Check sheet for the modelled part. Datum: model origin and axes. Units: mm. A direction names the side the tool comes from. Give positions to 0.01 mm unless a question says otherwise; leave off trailing zeros. Write each loop counter-clockwise with the first axis right and the second up, starting at its lowest first coordinate (ties: lowest second). Pieces come first, ordered by that corner, then holes. Notation, with made-up numbers: M 65,-20.75 L 85,-20.75 A21 ccw 85,12.25 Z; hole C 51.25,-20.5 d4. An arc over 180 degrees is marked long. One line per item, written item: value. Start each with the question number.
Autodesk Inventor part; units mm, degrees
ref_plane "Start plane" through (0, 0, 4.5945) normal (0, 0, 1) x (1, 0, 0)
ref_plane "End plane" through (0, 0, 785.2713) normal (0, 0, 1) x (1, 0, 0)
ref_plane "Work Plane4" through (0, 8.5964, 774.6227) normal (0, -0.4912, 0.871) x (1, 0, 0)
ref_plane "Start plane" through (0, 0, 4.5945) normal (0, 0, 1) x (1, 0, 0)
ref_plane "End plane" through (0, 0, 785.2713) normal (0, 0, 1) x (1, 0, 0)
sketch "Sketch" plane through (0, 0, 0) normal (0, 0, 1) x (1, 0, 0)
  line L0 (-17.5, -14.3) -> (-17.5, 14.3)
  line L1 (-14.3, 17.5) -> (14.3, 17.5)
  line L2 (17.5, 14.3) -> (17.5, -14.3)
  line L3 (14.3, -17.5) -> (-14.3, -17.5)
  arc A0 (-17.5, -14.3) -> (-14.3, -17.5) centre (-14.3, -14.3) ccw
  arc A1 (-14.3, 17.5) -> (-17.5, 14.3) centre (-14.3, 14.3) ccw
  arc A2 (17.5, 14.3) -> (14.3, 17.5) centre (14.3, 14.3) ccw
  arc A3 (14.3, -17.5) -> (17.5, -14.3) centre (14.3, -14.3) ccw
  arc A4 (-14.3, 15.9) -> (-15.9, 14.3) centre (-14.3, 14.3) ccw
  line L4 (-14.3, 15.9) -> (14.3, 15.9)
  arc A5 (15.9, 14.3) -> (14.3, 15.9) centre (14.3, 14.3) ccw
  line L5 (15.9, 14.3) -> (15.9, -14.3)
  arc A6 (14.3, -15.9) -> (15.9, -14.3) centre (14.3, -14.3) ccw
  line L6 (14.3, -15.9) -> (-14.3, -15.9)
  arc A7 (-15.9, -14.3) -> (-14.3, -15.9) centre (-14.3, -14.3) ccw
  line L7 (-15.9, -14.3) -> (-15.9, 14.3)
  line L8 (0, 25.4278) -> (0, -25.4278) construction
  line L9 (-25.4278, 0) -> (25.4278, 0) construction
  dimension "d7" = 3.2
  dimension "d10" = 35
  dimension "d11" = 35
  dimension "d12" = 1.6
  dimension "d15" = 17.5
  dimension "d16" = 17.5
extrude "Body" add sketch "Sketch" along normal up to surface (780.6769 mm away) from surface at 4.5945
sketch "Sketch3" plane through (0, 0, 0) normal (0, 0, 1) x (1, 0, 0)
  line L0 (0, 0) -> (10, 0)
ref_plane "Work Plane3" through (0, 0, 0) normal (0, -1, 0) x (1, 0, 0)
sketch "Sketch4" plane through (0, 0, 0) normal (0, -1, 0) x (1, 0, 0)
  line L0 (-2, 4.5945) -> (12, 4.5945)
  line L1 (-2, 785.2713) -> (12, 785.2713)
  dimension "d18" = 780.6769
ref_plane "Work Plane4" through (0, 8.5964, 774.6227) normal (0, -0.4912, 0.871) x (1, 0, 0)
split "Split1" plane through (0, 8.5964, 774.6227) removes the side toward (0, -0.4912, 0.871)
ref_plane "Work Plane5" through (0, -15.2431, 781.2694) normal (0, 0.871, 0.4912) x (1, 0, 0)
split "Split2" plane through (0, -15.2431, 781.2694) removes the side toward (0, 0.871, 0.4912)
ref_plane "Work Plane6" through (0, -8.5964, 15.2431) normal (0, 0.4912, -0.871) x (1, 0, 0)
split "Split3" plane through (0, -8.5964, 15.2431) removes the side toward (0, 0.4912, -0.871)
ref_plane "Work Plane7" through (0, -355.4612, 665.9277) normal (0, -0.871, -0.4912) x (1, 0, 0)
split "Split4" plane through (0, -355.4612, 665.9277) removes the side toward (0, -0.871, -0.4912)
equation "\"d7\" = G_IR"
equation "\"d10\" = G_H"
equation "\"d11\" = G_W"
equation "\"d12\" = G_T"
equation "\"d15\" = 0.5 * d10"
equation "\"d16\" = 0.5 * d11"
equation "\"d3\" = G_L"
equation "\"G_W\" = 35"
equation "\"G_H\" = 35"
equation "\"G_T\" = 1.6"
equation "\"G_IR\" = 3.2"
equation "\"G_L\" = d18"
equation "\"G_OFFSET_START\" = -4.59446"
equation "\"G_OFFSET_END\" = -4.59446"
equation "\"d13\" = -G_OFFSET_START"
equation "\"d14\" = G_OFFSET_END + B_L"
equation "\"B_L\" = 789.86581"
properties part number "AS 1163 - C350L0 35x35x1.6 SHS - 780.677" material "Steel, Mild"
1) Draft check along Y on faces 1 (the flat face through (-17.5, 0, 390)), 2 (the flat face through (0, -17.5, 408)), 3 (the flat face through (0, 17.5, 372)), 4 (the flat face through (0, -15.9, 407)). Enter one of: released by +Y, released by -Y, zero draft, split by the parting line, or undercut.
2) Gauge pin test, flat end, axial feed: pin 1 (12 mm diameter, centred on x = 4.5, y = -7, fed in from -Z). Record the tip position at first contact, or that the pin passes through.
3) Material ranges on L1, parallel to Y at x = 7.5, z = 73; L2, parallel to X at y = -15.5, z = 149.5, recorded low to high. Write a range as from..to.
4) Cross-section at C-C (y = 0.5). Record the boundary of the cut face in (x, z).
5) Cross-section at A-A (x = 0). Record the boundary of the cut face in (y, z), plus the area to 3 significant figures.
6) Cross-section at B-B (z = 653). Record the boundary of the cut face in (x, y), plus the area to 3 significant figures.
7) Tool access check on faces 5 (the flat face through (15.9, 0, 390)), 6 (the flat face through (17.5, 0, 390)). Record the directions out of +Z, -Z, +X, -X, +Y, -Y that give a thin tool (end or side, any length) a straight path to the whole face; none if there is none.
Data:
1. face 1: zero draft
1. face 2: released by -Y
1. face 3: released by +Y
1. face 4: undercut
2. pin 1: passes through
3. L1: y = -17.5..-15.9, 15.9..17.5
3. L2: x = -17.27..-15.36, 15.36..17.27
4. outline: M -17.5,34.73 L -15.9,34.73 L -15.9,753.35 L -17.5,753.35 Z; M 15.9,34.73 L 17.5,34.73 L 17.5,753.35 L 15.9,753.35 Z
5. outline: M -17.5,66.65 L -15.9,63.81 L -15.9,760.81 L -17.5,759.91 Z; M 15.9,29.06 L 17.5,29.96 L 17.5,723.21 L 15.9,726.05 Z
5. area: 2,220 mm2
6. outline: M -17.5,-14.3 A3.2 ccw -14.3,-17.5 L 14.3,-17.5 A3.2 ccw 17.5,-14.3 L 17.5,14.3 A3.2 ccw 14.3,17.5 L -14.3,17.5 A3.2 ccw -17.5,14.3 Z; hole M -15.9,-14.3 A1.6 ccw -14.3,-15.9 L 14.3,-15.9 A1.6 ccw 15.9,-14.3 L 15.9,14.3 A1.6 ccw 14.3,15.9 L -14.3,15.9 A1.6 ccw -15.9,14.3 Z
6. area: 207 mm2
7. face 5: +Z, -Z
7. face 6: +Z, -Z, +X, +Y, -Y
